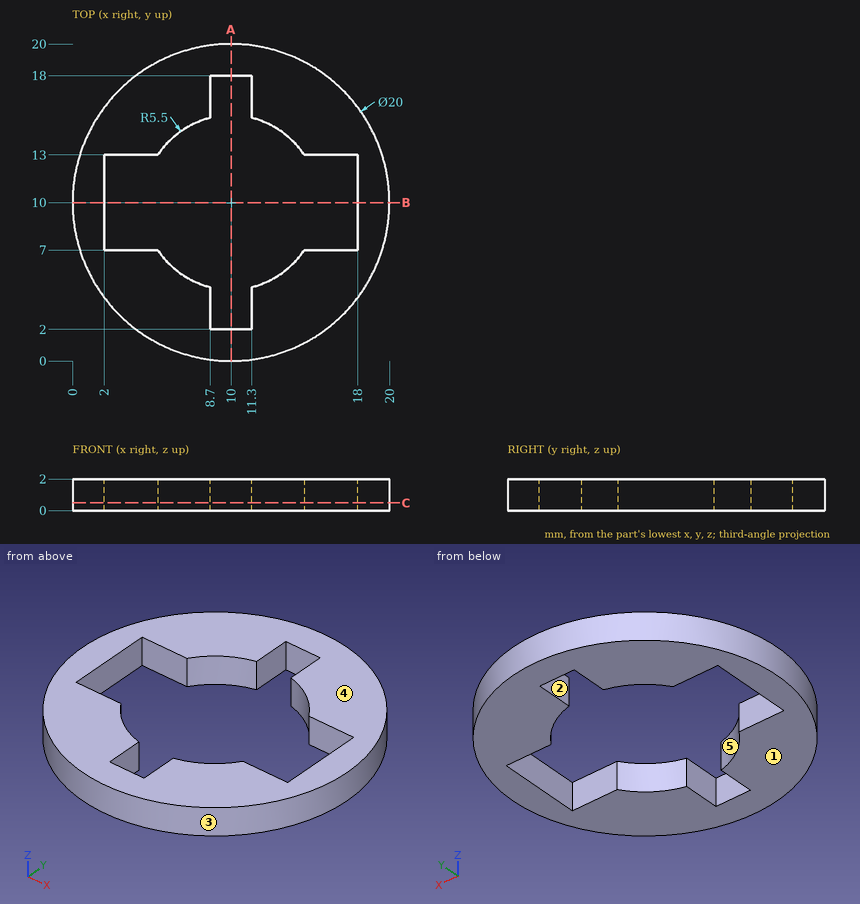
Study the drawing (mm; zero at the part's minimum x, y, z) and answer. A direction names the side the tool comes from. Round coordinates to 2 decimals unless told otherwise and drop trailing zeros. Loops run counter-clockwise (first coordinate to the right, second up) from the corner with the lowest first, then second, coordinate; pieces in that order, holes last. Notation, with made-up numbers: M 4.25,60 L 55.25,60 A12 ccw 55.25,69 Z; hole C -39,77 d10. An arc over 180 degrees is marked long. One line per question, with ' | ' between items.
Q1. Find section C-C, the plane z = 0.5. Give the vertices of the cut face in (x, y), then the cut area to 3 significant figures.
Conclusion:
outline: C 10,10 d20; hole M 2,7 L 5.39,7 A5.5 ccw 8.7,4.66 L 8.7,2 L 11.3,2 L 11.3,4.66 A5.5 ccw 14.61,7 L 18,7 L 18,13 L 14.61,13 A5.5 ccw 11.3,15.34 L 11.3,18 L 8.7,18 L 8.7,15.34 A5.5 ccw 5.39,13 L 2,13 Z | area: 172 mm2
Q2. Consider line 1 along X through (y, z) = (4, 0.8); line 2 along X through (y, z) = (7.75, 0.3); line 3 along Y through (x, z) = (4, 1.2). Determine where each line is inside the solid, lowest interval first. Write a range as from..to.
Conclusion:
line 1: x = 2..8.7, 11.3..18 | line 2: x = 0.26..2, 18..19.74 | line 3: y = 2..7, 13..18
Q3. Each of these flat-tipped pins is pushed along its axis until it touches: pin 1 Ø0.6 at (y, z) = (16.5, 1.5) entering from +X; pin 2 Ø0.6 at (y, z) = (16.5, 0.5) entering from -X; pin 3 Ø1 at (y, z) = (17, 1) entering from -X. Where does it stop, or does it pass through?
Conclusion:
pin 1: stops at x = 17.85 | pin 2: stops at x = 2.15 | pin 3: stops at x = 2.4
Q4. Find section A-A, the plane x = 10. Give the vertices of the cut face in (y, z).
Conclusion:
outline: M 0,0 L 2,0 L 2,2 L 0,2 Z; M 18,0 L 20,0 L 20,2 L 18,2 Z
Q5. A tool of negligible diameter and unlimited length cuts with its end or side. For the marked faces 4 and 5, from which of +Z, -Z, +X, -X, +Y, -Y can it reach the whole face along a straight path? Write none if from no direction.
Conclusion:
face 4: +Z, +X, -X, +Y, -Y | face 5: +Z, -Z
Q6. The mould has two halves that part along Y. Classify the marked faces 1, 2 and 3: +Y half, -Y half, draft (parallel to the pull), parting line (faces both ways), or undercut.
Conclusion:
face 1: draft | face 2: undercut | face 3: parting line
